from build123d import *

# Parameters (mm, degrees)
SKICA1_W                    = 67
SKICA1_H                    = 50
P_IDAT_VYSUNUT_M1_DEPTH     = 3
ODEBRAT_VYSUNUT_M1_DEPTH    = 1
SKICA3_W                    = 8
SKICA3_H                    = 8
ODEBRAT_VYSUNUT_M2_DEPTH    = 4
VYSUNOUT_TENKOST_NN_1_DEPTH = 1
VYSUNOUT_TENKOST_NN_2_DEPTH = 5
SKICA6_W                    = 12
SKICA6_H                    = 4
ODEBRAT_VYSUNUT_M3_DEPTH    = 4
ODEBRAT_VYSUNUT_M4_DEPTH    = 1
P_IDAT_START                = -1
SKICA8_W                    = 2
SKICA8_H                    = 2
P_IDAT_VYSUNUT_M2_DEPTH     = 1
ODEBRAT_VYSUNUT_M5_DEPTH    = 1
SKICA10_W                   = 1.6
SKICA10_H                   = 2.4
SKICA10_H_2                 = 1.6
P_IDAT_VYSUNUT_M3_DEPTH     = 1


with BuildPart() as part:
    # Skica1 → Přidat vysunutím1 (new body)
    with BuildSketch(Plane.XY):
        Rectangle(SKICA1_W, SKICA1_H)
    extrude(amount=P_IDAT_VYSUNUT_M1_DEPTH)

    # Skica2 → Odebrat vysunutím1 (cut)
    with BuildSketch(Plane.XY.offset(3)):
        Polygon((-25.5, -22), (-30.5, -17), (-30.5, 17), (-25.5, 22), (25.5, 22), (30.5, 17), (30.5, -17), (25.5, -22), align=None)
    extrude(amount=-ODEBRAT_VYSUNUT_M1_DEPTH, mode=Mode.SUBTRACT)

    # Skica3 → Odebrat vysunutím2 (cut, through all)
    with BuildSketch(Plane(origin=(0, 0, 0), x_dir=(-1, 0, 0), z_dir=(0, 0, -1))):
        with Locations((20, -3)):
            Rectangle(SKICA3_W, SKICA3_H)
        with Locations((-20, -3)):
            Rectangle(SKICA3_W, SKICA3_H)
        Polygon((25.5, -25), (-25.5, -25), (-25.5, -12), (-12, -12), (-12, 15), (12, 15), (12, -12), (25.5, -12), align=None)
    extrude(amount=-ODEBRAT_VYSUNUT_M2_DEPTH, mode=Mode.SUBTRACT)

    # Skica4 → Vysunout tenkostěnný1 (add)
    with BuildSketch(Plane.XY.offset(2)):
        Polygon((-12, -12), (-12, 15), (12, 15), (12, -12), (13, -12), (13, 16), (-13, 16), (-13, -12), align=None)
    extrude(amount=VYSUNOUT_TENKOST_NN_1_DEPTH)

    # Skica5 → Vysunout tenkostěnný2 (add)
    with BuildSketch(Plane(origin=(0, 0, 0), x_dir=(-1, 0, 0), z_dir=(0, 0, -1))):
        Polygon((-25.5, -25), (-33.5, -25), (-33.5, 25), (33.5, 25), (33.5, -25), (25.5, -25), (25.5, -26), (34.5, -26), (34.5, 26), (-34.5, 26), (-34.5, -26), (-25.5, -26), align=None)
    extrude(amount=-VYSUNOUT_TENKOST_NN_2_DEPTH)

    # Skica6 → Odebrat vysunutím3 (cut, through all)
    with BuildSketch(Plane.XY.offset(2)):
        with Locations((0, 24)):
            Rectangle(SKICA6_W, SKICA6_H)
    extrude(amount=ODEBRAT_VYSUNUT_M3_DEPTH, mode=Mode.SUBTRACT)

    # Skica7 → Odebrat vysunutím4 (cut)
    with BuildSketch(Plane(origin=(0, 0, 0), x_dir=(-1, 0, 0), z_dir=(0, 0, -1))):
        Polygon((-28.75, 22), (-26.75, 22), (-26.75, 21), (-25.75, 21), (-25.75, 16), (-20.75, 16), (-20.75, 21), (-19.75, 21), (-19.75, 22), (-17.75, 22), (-17.75, 21), (-16.75, 21), (-16.75, 14), (-15.75, 14), (-15.75, 8), (-16.75, 8), (-16.75, 7), (-17.75, 7), (-17.75, 6), (-18.75, 6), (-18.75, 5), (-27.75, 5), (-27.75, 6), (-28.75, 6), (-28.75, 7), (-29.75, 7), (-29.75, 8), (-30.75, 8), (-30.75, 14), (-29.75, 14), (-29.75, 21), (-28.75, 21), align=None)
        Polygon((18.75, 6), (18.75, 5), (27.75, 5), (27.75, 6), (28.75, 6), (28.75, 7), (29.75, 7), (29.75, 8), (30.75, 8), (30.75, 14), (29.75, 14), (29.75, 21), (28.75, 21), (28.75, 22), (26.75, 22), (26.75, 21), (25.75, 21), (25.75, 16), (20.75, 16), (20.75, 21), (19.75, 21), (19.75, 22), (17.75, 22), (17.75, 21), (16.75, 21), (16.75, 14), (15.75, 14), (15.75, 8), (16.75, 8), (16.75, 7), (17.75, 7), (17.75, 6), align=None)
    extrude(amount=-ODEBRAT_VYSUNUT_M4_DEPTH, mode=Mode.SUBTRACT)

    # Skica8 → Přidat vysunutím2 (add)
    with BuildSketch(Plane(origin=(0, 0, 0), x_dir=(-1, 0, 0), z_dir=(0, 0, -1)).offset(P_IDAT_START)):
        with Locations((-26.75, 11)):
            Rectangle(SKICA8_W, SKICA8_H)
        with Locations((-19.75, 11)):
            Rectangle(SKICA8_W, SKICA8_H)
        Polygon((-23.75, 10), (-22.75, 10), (-22.75, 9), (-21.75, 9), (-21.75, 8), (-24.75, 8), (-24.75, 9), (-23.75, 9), align=None)
        Polygon((24.75, 9), (23.75, 9), (23.75, 10), (22.75, 10), (22.75, 9), (21.75, 9), (21.75, 8), (24.75, 8), align=None)
        with Locations((26.75, 11)):
            Rectangle(SKICA8_W, SKICA8_H)
        with Locations((19.75, 11)):
            Rectangle(SKICA8_W, SKICA8_H)
    extrude(amount=P_IDAT_VYSUNUT_M2_DEPTH)

    # Skica9 → Odebrat vysunutím5 (cut)
    with BuildSketch(Plane(origin=(0, 0, 0), x_dir=(-1, 0, 0), z_dir=(0, 0, -1))):
        Polygon((-11.2, 23.3), (-9.6, 23.3), (-9.6, 19.3), (-8.8, 19.3), (-8.8, 21.7), (-8, 21.7), (-8, 19.3), (-7.2, 19.3), (-7.2, 23.3), (-5.6, 23.3), (-5.6, 18.5), (-6.4, 18.5), (-6.4, 17.7), (-8, 17.7), (-8, 18.5), (-8.8, 18.5), (-8.8, 17.7), (-10.4, 17.7), (-10.4, 18.5), (-11.2, 18.5), align=None)
        Polygon((-4.8, 23.3), (-3.2, 23.3), (-3.2, 20.9), (-1.6, 20.9), (-1.6, 23.3), (0, 23.3), (0, 17.7), (-1.6, 17.7), (-1.6, 20.1), (-3.2, 20.1), (-3.2, 17.7), (-4.8, 17.7), align=None)
        Polygon((1.6, 23.3), (4.8, 23.3), (4.8, 22.5), (5.6, 22.5), (5.6, 18.5), (4.8, 18.5), (4.8, 17.7), (1.6, 17.7), (1.6, 18.5), (0.8, 18.5), (0.8, 22.5), (1.6, 22.5), align=None)
        Polygon((6.4, 23.3), (10.4, 23.3), (10.4, 22.5), (11.2, 22.5), (11.2, 20.9), (10.4, 20.9), (10.4, 20.1), (8, 20.1), (8, 17.7), (6.4, 17.7), align=None)
    extrude(amount=-ODEBRAT_VYSUNUT_M5_DEPTH, mode=Mode.SUBTRACT)

    # Skica10 → Přidat vysunutím3 (add)
    with BuildSketch(Plane(origin=(0, 0, 0), x_dir=(-1, 0, 0), z_dir=(0, 0, -1)).offset(P_IDAT_START)):
        with Locations((3.2, 20.5)):
            Rectangle(SKICA10_W, SKICA10_H)
        with Locations((8.8, 21.7)):
            Rectangle(SKICA10_W, SKICA10_H_2)
    extrude(amount=P_IDAT_VYSUNUT_M3_DEPTH)


solid = part.part
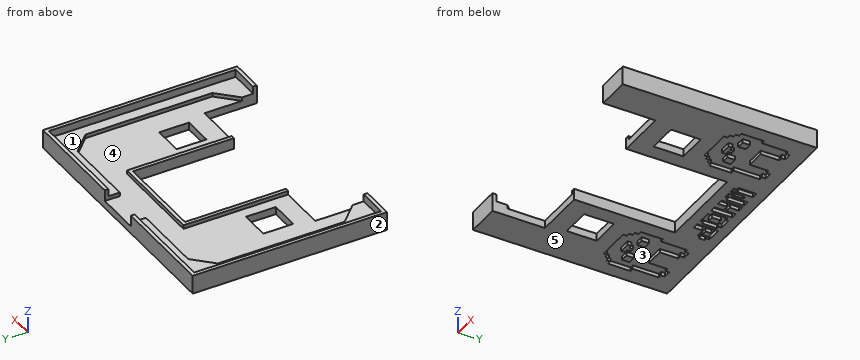
The model under review builds one solid part; all positions refer to its coordinate system, in mm. Face numbers are marked on the shaded views. A direction names the side the tool comes from. Round coordinates to 2 decimals unless told otherwise and drop trailing zeros. Loops run counter-clockwise (first coordinate to the right, second up) from the corner with the lowest first, then second, coordinate; pieces in that order, holes last. Notation, with made-up numbers: M 65,-1 L 117,-1 A31 ccw 117,25 Z; hole C 53,74.5 d9. An arc over 180 degrees is marked long. Answer as a JSON object with one key per item and string values.
Item 1: We need section C-C, the plane y = -20.5. State the section outline as (x, z) points.
Check sheet entries:
{"outline": "M -34.5,0 L -25.5,0 L -25.5,2 L -27,2 L -27,3 L -33.5,3 L -33.5,5 L -34.5,5 Z; M 25.5,0 L 34.5,0 L 34.5,5 L 33.5,5 L 33.5,3 L 27,3 L 27,2 L 25.5,2 Z"}
Item 2: Clearance check with flat-ended pins moving along their axes: P1, Ø0.5, axis at x = -20.5, z = 0.5, coming from the -Y side; P2, Ø21, axis at x = -3, y = 1, coming from the +Z side; P3, Ø2, axis at x = -25, y = -3.5, coming from the -Z side; P4, Ø3, axis at x = 4.5, z = 2.5, coming from the -Y side. State where each tip first meets the part, or that it passes through.
Check sheet entries:
{"P1": "y = -12", "P2": "z = 3", "P3": "z = 0", "P4": "y = 15"}
Item 3: Tool access review of the marked faces 1 and 2: name each direction out of +Z, -Z, +X, -X, +Y, -Y from which nothing blocks a thin tool from reaching the whole face with its end or side.
Check sheet entries:
{"face 1": "+Z", "face 2": "+Z, -Z, -X, +Y, -Y"}
Item 4: The part is to be moulded in two halves that separate along Y. For the marked faces 3, 4 and 5, say which applies: +Y half, -Y half, draft (parallel to the pull), parting line (faces both ways), or undercut.
Check sheet entries:
{"face 3": "undercut", "face 4": "undercut", "face 5": "draft"}
Item 5: We need section B-B, the plane z = 3.75. State the section outline as (x, y) points.
Check sheet entries:
{"outline": "M -34.5,-26 L -25.5,-26 L -25.5,-25 L -33.5,-25 L -33.5,25 L -6,25 L -6,26 L -34.5,26 Z; M 6,25 L 33.5,25 L 33.5,-25 L 25.5,-25 L 25.5,-26 L 34.5,-26 L 34.5,26 L 6,26 Z"}
Item 6: We need section D-D, the plane x = 15. State the section outline as (y, z) points.
Check sheet entries:
{"outline": "M -12,0 L 26,0 L 26,5 L 25,5 L 25,3 L 22,3 L 22,2 L -12,2 Z"}
Item 7: We need section A-A, the plane y = -5. State the section outline as (x, z) points, and give its area (3 significant figures).
Check sheet entries:
{"outline": "M -34.5,0 L -24,0 L -24,2 L -30.5,2 L -30.5,3 L -33.5,3 L -33.5,5 L -34.5,5 Z; M -16,0 L -12,0 L -12,3 L -13,3 L -13,2 L -16,2 Z; M 12,0 L 16,0 L 16,2 L 13,2 L 13,3 L 12,3 Z; M 24,0 L 34.5,0 L 34.5,5 L 33.5,5 L 33.5,3 L 30.5,3 L 30.5,2 L 24,2 Z", "area": "72.0 mm2"}
Item 8: For line 1 along X through (y, z) = (-2, 2.2); line 2 along X through (y, z) = (-10.5, 4); line 3 along X through (y, z) = (-9.5, 1.2), list the stretches that pass through material, from the lowest coordinate up.
Check sheet entries:
{"line 1": "-34.5 to -30.5, -13 to -12, 12 to 13, 30.5 to 34.5", "line 2": "-34.5 to -33.5, 33.5 to 34.5", "line 3": "-34.5 to -12, 12 to 34.5"}
